from build123d import *

# Parameters (mm, degrees)
F2_DEPTH = 25.4
F3_DEPTH = 12.7


# Not quite as in the source:
# - a length typed as a fraction of an inch, garbled in the dataset ("3 / 203.2 mm" for 3/8 in), is restored


with BuildPart() as f2:
    # F1 (on face) → F2 (new body)
    with BuildSketch(Plane.XY):
        Polygon((-29.84200418, 14.5122259855), (128.3614784479, -24.7320532799), (0, 14.5122259855), align=None)
    extrude(amount=F2_DEPTH)

    # F3 (add): a face of the model
    f3_faces = [f2.faces().sort_by_distance(p)[0] for p in [
        (49.259737134, -5.1099136472, 12.7),
    ]]
    extrude(f3_faces, amount=F3_DEPTH)


solid = f2.part
The listing builds one solid part. Answer for the finished solid, in the listing's coordinates (mm). Give positions to 0.01 mm unless a question says otherwise; leave off trailing zeros. Order: outer loops, then holes, each group sorted by start corner. A loop starts at its lowest first (then second) coordinate and runs counter-clockwise, first axis right, second up. Notation, with made-up numbers: (27.25, 65) - (38.25, 65) arc R36 ccw to (38.25, 104) - close; hole circle Ø7 at (-33.5, -26.75). An arc over 180 degrees is marked (long way). Answer as CSV lines item,"result".
Q1. Straight lines are drawn through the part: L1, parallel to Y at x = -8.5, z = 22.75; L2, parallel to Y at x = 113, z = 20.75. For each, find the intervals that lie inside material, in ascending order.
Answer key:
L1,"y = -3.87 to 14.51"
L2,"y = -34.01 to -20.04"
Q2. A cutting plane is placed at A-A, the plane z = 14.25. Determine the outline of the cut face in (x, y), and give its area (3 significant figures).
Answer key:
outline,"(-32.9, 2.19) - (125.3, -37.06) - (128.36, -24.73) - (0, 14.51) - (-29.84, 14.51) - close"
area,"2,660 mm^2"
Q3. Each of these flat-tipped pins is pushed along its axis until it touches: pin 1 Ø3 at (x, z) = (51.5, 3.5) entering from -Y; pin 2 Ø1 at (x, z) = (47, 5) entering from -Y. Where does it stop, or does it pass through?
Answer key:
pin 1,"stops at y = -19.12"
pin 2,"stops at y = -17.76"
Q4. A cutting plane is placed at C-C, the plane y = -9.5. Determine the outline of the cut face in (x, z).
Answer key:
outline,"(14.21, 0) - (78.54, 0) - (78.54, 25.4) - (14.21, 25.4) - close"
Q5. A cutting plane is placed at B-B, the plane x = 89. Determine the outline of the cut face in (y, z).
Answer key:
outline,"(-28.05, 0) - (-12.7, 0) - (-12.7, 25.4) - (-28.05, 25.4) - close"
